Verification items for the finished model (mm, model axes). Give positions to 0.01 mm unless a question says otherwise; leave off trailing zeros. Loops run counter-clockwise (first coordinate to the right, second up) from the corner with the lowest first, then second, coordinate; pieces in that order, holes last. Notation, with made-up numbers: M 65,88.5 L 78,88.5 A22 cw 78,117.5 Z; hole C 31.5,60.25 d9. An arc over 180 degrees is marked long. Answer in a Markdown table with one row per item.
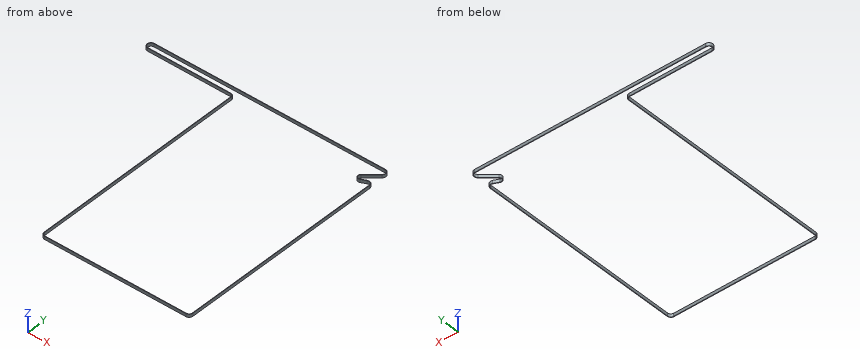
```python
from build123d import *

# Parameters (mm, degrees)
SKETCH3_W = 6
SKETCH3_H = 1


with BuildPart() as part:
    # Sweep1: sweep along a path in Sketch2
    with BuildLine(Plane.XY) as sweep1_path:
        Line((7.533930162, -5.559792976), (17.781318169, -0.889445417))
        ThreePointArc((17.781318169, -0.889445417), (23.99309151, -1.337216564), (26.976988544, -6.803749792))
        Line((26.976988544, -6.803749792), (26.99999999, -412.150308572))
        ThreePointArc((26.99999999, -412.150308572), (25.095317263, -416.747748302), (20.497151225, -418.650676952))
        Line((20.497151225, -418.650676952), (-260.786858168, -418.527397737))
        ThreePointArc((-260.786858168, -418.527397737), (-265.378263623, -416.625531469), (-267.28400405, -412.035732696))
        Line((-267.28400405, -412.035732696), (-267.834014416, 16.920435322))
        ThreePointArc((-267.834014416, 16.920435322), (-269.61983276, 21.229266015), (-273.925552043, 23.022573168))
        Line((-273.925552043, 23.022573168), (-439.549241213, 23.522898593))
        ThreePointArc((-439.549241213, 23.522898593), (-446.029600051, 30.031464399), (-439.53205031, 36.522868475))
        Line((-439.53205031, 36.522868475), (20.497555424, 36.695880369))
        ThreePointArc((20.497555424, 36.695880369), (26.58757217, 32.474359504), (24.7659723, 25.291649968))
        Line((24.7659723, 25.291649968), (0.989986039, 4.609977009))
        ThreePointArc((0.989986039, 4.609977009), (-0.138167108, -3.306257517), (7.533930162, -5.559792976))
    # Sketch3 → Sweep1 (sweep)
    with BuildSketch(Plane(origin=(0, 0, 0), x_dir=(0, 0, -1), z_dir=(1, 0, 0))):
        with Locations((0, 37.195880369)):
            Rectangle(SKETCH3_W, SKETCH3_H)
    sweep(path=sweep1_path.line)


solid = part.part
```
Item 1: Sectioned sample at B-B (x = -325). Record the cut outline in (y, z).
Reported:
| item | result |
|---|---|
| outline | M 22.17,-3 L 23.17,-3 L 23.17,3 L 22.17,3 Z; M 36.57,-3 L 37.57,-3 L 37.57,3 L 36.57,3 Z |
Item 2: Scan lines: L1, parallel to Y at x = -238.5, z = 1.5; L2, parallel to Y at x = -94, z = 2.75; L3, parallel to X at y = -36, z = 1. Record each from-to range of solid material in increasing order. Write a range as [from, to].
Reported:
| item | result |
|---|---|
| L1 | y = [-419.54, -418.54], [36.61, 37.61] |
| L2 | y = [-419.61, -418.61], [36.66, 37.66] |
| L3 | x = [-268.77, -267.77], [26.99, 27.99] |
Item 3: Sectioned sample at C-C (y = -326.5). Record the cut outline in (x, z).
Reported:
| item | result |
|---|---|
| outline | M -268.4,-3 L -267.4,-3 L -267.4,3 L -268.4,3 Z; M 27,-3 L 28,-3 L 28,3 L 27,3 Z |
Item 4: Sectioned sample at A-A (z = 1.15). Record the cut outline in (x, y).
Reported:
| item | result |
|---|---|
| outline | M -439.55,22.52 L -273.93,22.01 A5.1 cw -268.84,16.92 L -268.29,-412.04 A7.51 ccw -260.79,-419.54 L 20.5,-419.66 A7.51 ccw 28.01,-412.15 L 27.98,-6.8 A7.51 ccw 17.36,0.03 L 7.12,-4.64 A5.1 cw 1.65,3.85 L 25.43,24.53 A7.51 ccw 20.5,37.7 L -439.53,37.53 A7.51 ccw Z; hole M -439.55,23.52 L -273.93,23.01 A6.1 cw -267.84,16.92 L -267.29,-412.04 A6.51 ccw -260.79,-418.54 L 20.5,-418.66 A6.51 ccw 27.01,-412.15 L 26.98,-6.8 A6.51 ccw 17.78,-0.88 L 7.53,-5.55 A6.1 cw 1,4.6 L 24.77,25.29 A6.51 ccw 20.5,36.7 L -439.53,36.53 A6.51 ccw Z |
Item 5: Go/stop test with flat-tipped pins: pin 1 (2 mm diameter, centred on x = -365.5, z = 0, fed in from +Y); pin 2 (3 mm diameter, centred on y = -317, z = 0.5, fed in from -X); pin 3 (1.8 mm diameter, centred on x = -268, z = 1, fed in from -Y). Record where each tip stops, or that it passes through.
Reported:
| item | result |
|---|---|
| pin 1 | stops at y = 37.56 |
| pin 2 | stops at x = -268.42 |
| pin 3 | stops at y = -416.09 |
